```python
from build123d import *

# Parameters (mm, degrees)
F1_DEPTH = 25


with BuildPart() as f1:
    # F0 (on Top) → F1 (new body)
    with BuildSketch(Plane.XY):
        with BuildLine():
            ThreePointArc((-55.021506, 32.166502), (-55.958015, 31.67005), (-56.33252, 30.678455))
            Line((-56.33252, 30.678455), (-56.33252, 1.5))
            ThreePointArc((-56.33252, 1.5), (-55.89318, 0.43934), (-54.83252, 0))
            Line((-54.83252, 0), (47.16748, 0))
            ThreePointArc((47.16748, 0), (48.228141, 0.43934), (48.66748, 1.5))
            Line((48.66748, 1.5), (48.66748, 51))
            ThreePointArc((48.66748, 51), (47.788801, 53.12132), (45.66748, 54))
            Line((45.66748, 54), (34.66748, 54))
            Line((34.66748, 54), (34.66748, 44))
            Line((34.66748, 44), (-6.117023, 38.210268))
            Line((-6.117023, 38.210268), (-6.117023, 32))
            Line((-6.117023, 32), (-20.117023, 32))
            Line((-20.117023, 32), (-20.117023, 36.599465))
            Line((-20.117023, 36.599465), (-55.021506, 32.166502))
        make_face()
    extrude(amount=F1_DEPTH)


solid = f1.part
```
Build history of the part. All positions in model axes, mm. A direction names the side the tool comes from. Coordinates: 2 decimals unless noted, no trailing zeros. Order: outer loops, then holes, each group sorted by start corner. A loop starts at its lowest first (then second) coordinate and runs counter-clockwise, first axis right, second up. Notation, with made-up numbers: M 28,-4 L 38,-4 A26 ccw 38,30 Z; hole C -7.5,71 d6. An arc over 180 degrees is marked long. One line per question, with ' | ' between items. Start each with the question number.
1. Cut at B-B (y = 47). Write the cut outline in (x, z), plus the area to 3 significant figures.
2. Cut at C-C (x = 7). Write the cut outline in (y, z).
3. Mould opens along X. For faces 1 (the face through (-20.117, 34, 12)), 2 (the face through (-5, 21, 25)), 3 (the face through (34.667, 49, 12)) say: +X half, -X half, draft (parallel to the pull), parting line (faces both ways), or undercut.
4. Flat gauge pins, fed straight in: P1, Ø5, axis at y = 49, z = 16, coming from the -X side; P2, Ø11, axis at x = -12.5, z = 7, coming from the +Y side; P3, Ø5, axis at y = 33.5, z = 7.5, coming from the -X side. Where does each tip first touch, or does it go through?
5. Cut at A-A (z = 18.5). Write the cut outline in (x, y).
6. Tool access for faces 4 (the face through (-37.325, 34.414, 12.325)), 5 (the face through (-13, 32, 12)): list every direction of +Z, -Z, +X, -X, +Y, -Y with a clear straight run to the whole face (end or side of a thin tool).
7. Wall check: line 1 along X through (y, z) = (46.5, 13.5); line 2 along Y through (x, z) = (-10.5, 18.25); line 3 along Y through (x, z) = (-34, 6.25). Give the ranges that are in metal, low to high. Write a range as [from, to].
The answers:
1) outline: M 34.67,0 L 48.67,0 L 48.67,25 L 34.67,25 Z | area: 350 mm2
2) outline: M 0,0 L 40.07,0 L 40.07,25 L 0,25 Z
3) face 1: undercut | face 2: draft | face 3: -X half
4) P1: stops at x = 34.67 | P2: stops at y = 32 | P3: stops at x = -56.3
5) outline: M -56.33,1.5 A1.5 ccw -54.83,0 L 47.17,0 A1.5 ccw 48.67,1.5 L 48.67,51 A3 ccw 45.67,54 L 34.67,54 L 34.67,44 L -6.12,38.21 L -6.12,32 L -20.12,32 L -20.12,36.6 L -55.02,32.17 A1.5 ccw -56.33,30.68 Z
6) face 4: +Z, -Z, -X, +Y | face 5: +Z, -Z, +Y
7) line 1: x = [34.67, 48.67] | line 2: y = [0, 32] | line 3: y = [0, 34.84]
